The model under review builds one solid part; all positions refer to its coordinate system, in mm. Face numbers are marked on the shaded views. Coordinates: 2 decimals unless noted, no trailing zeros. Order: outer loops, then holes, each group sorted by start corner. A loop starts at its lowest first (then second) coordinate and runs counter-clockwise, first axis right, second up. Notation, with made-up numbers: (3, 25.25) -> (49, 25.25) arc R23 ccw to (49, 57.25) -> close; hole circle Ø1 at (71.25, -13). An arc over 180 degrees is marked (long way). Use one line per item in the form item = value.
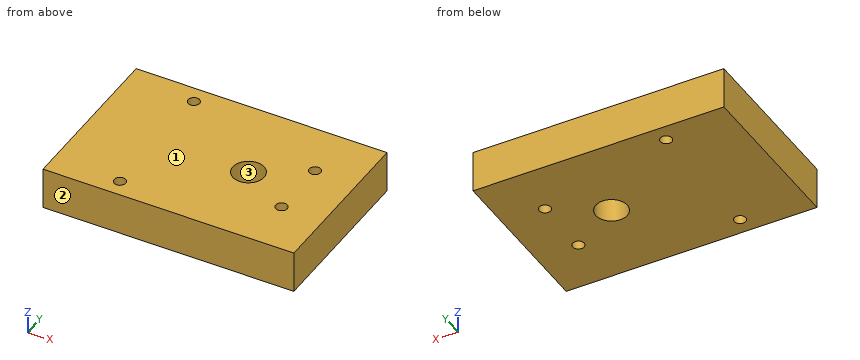
from build123d import *

# Parameters (mm, degrees)
F0_W     = 76.2
F0_H     = 50.8
F1_DEPTH = 12.7
F3_D     = 9.525
F5_D     = 3.5052


with BuildPart() as f1:
    # F0 (on Top) → F1 (new body)
    with BuildSketch(Plane.XY):
        with Locations((-10.16, 0)):
            Rectangle(F0_W, F0_H)
    extrude(amount=F1_DEPTH)

    # F3 (through all)
    with Locations(Plane.XY.offset(12.7)):
        with Locations((0, 0)):
            Hole(F3_D / 2)

    # F5 (through all)
    with Locations(Plane.XY.offset(12.7)):
        with Locations((15.1384, 9.1186), (15.1384, -9.1186), (-27.813, 20.1676), (-27.813, -20.1676)):
            Hole(F5_D / 2)


solid = f1.part
Item 1: We need section D-D (x = -28). Write out the cut boundary in (y, z) (3 decimals), plus the area to 3 significant figures.
Results found:
outline = (-25.4, 0) -> (-21.91, 0) -> (-21.91, 12.7) -> (-25.4, 12.7) -> close; (-18.425, 0) -> (18.425, 0) -> (18.425, 12.7) -> (-18.425, 12.7) -> close; (21.91, 0) -> (25.4, 0) -> (25.4, 12.7) -> (21.91, 12.7) -> close
area = 557 mm²
Item 2: Draft analysis for pull direction Y (two halves, no side actions). For the marked faces 1, 2 and 3, state which applies: released by +Y, released by -Y, zero draft, split by the parting line, or undercut.
Results found:
face_1 = zero draft
face_2 = released by -Y
face_3 = undercut
Item 3: We need section B-B (y = 0). Write out the cut boundary in (x, z).
Results found:
outline = (-48.26, 0) -> (-4.76, 0) -> (-4.76, 12.7) -> (-48.26, 12.7) -> close; (4.76, 0) -> (27.94, 0) -> (27.94, 12.7) -> (4.76, 12.7) -> close
Item 4: We need section A-A (x = 0). Write out the cut boundary in (y, z).
Results found:
outline = (-25.4, 0) -> (-4.76, 0) -> (-4.76, 12.7) -> (-25.4, 12.7) -> close; (4.76, 0) -> (25.4, 0) -> (25.4, 12.7) -> (4.76, 12.7) -> close
Item 5: Clearance check with flat-ended pins moving along their axes: pin 1 (2 mm diameter, centred on x = 15.14, y = 9.12, fed in from +Z); pin 2 (5.5 mm diameter, centred on x = -27.81, y = -20.17, fed in from -Z). State where each tip first meets the part, or that it passes through.
Results found:
pin_1 = through
pin_2 = 0
Item 6: We need section C-C (z = 2.5). Write out the cut boundary in (x, y) (1 decimal).
Results found:
outline = (-48.3, -25.4) -> (27.9, -25.4) -> (27.9, 25.4) -> (-48.3, 25.4) -> close; hole circle Ø3.5 at (-27.8, -20.2); hole circle Ø3.5 at (-27.8, 20.2); hole circle Ø9.5 at (0, 0); hole circle Ø3.5 at (15.1, -9.1); hole circle Ø3.5 at (15.1, 9.1)
Item 7: To check wall thickness, follow L1, parallel to Y at x = 0, z = 6.5; L2, parallel to Y at x = -3, z = 9; L3, parallel to X at y = 10, z = 11.25. State the ranges of each line that lie inside material, in increasing order. Write a range as from..to.
Results found:
L1 = -25.4..-4.76, 4.76..25.4
L2 = -25.4..-3.7, 3.7..25.4
L3 = -48.26..13.62, 16.65..27.94
